Geometry: final body of the model. Coordinates: model frame, mm. A direction names the side the tool comes from. Round coordinates to 2 decimals unless told otherwise and drop trailing zeros. Loops run counter-clockwise (first coordinate to the right, second up) from the corner with the lowest first, then second, coordinate; pieces in that order, holes last. Notation, with made-up numbers: (83, 37) - (125, 37) arc R28 ccw to (125, 55) - close; hole circle Ø11 at (16.5, 55). An arc over 180 degrees is marked (long way). Write item = value, one per line. Start each with the question number.
Item 1: Section D-D (z = 12). Return loops of the section in (x, y).
Item 2: First-contact query: pin 1 (2 mm diameter, centred on y = -29.5, z = 12, fed in from -X); pin 2 (9 mm diameter, centred on y = -0.5, z = -4, fed in from -X); pin 3 (1.5 mm diameter, centred on y = 29.5, z = -12, fed in from +X). Flat tips, straight axial feed; report the tip coordinate or a pass-through.
Item 3: Section A-A (x = -23). Return loops of the section in (y, z).
Item 4: Access query for faces 5 (the flat face through (-14, 6, 12)), 6 (the flat face through (0, 32.5, 0)), 7 (the cylindrical face through (28.5, 23.5, 0.1)). Directions: +Z, -Z, +X, -X, +Y, -Y. A direction counts if a zero-diameter tool reaches every point of the face in a straight line with its end or side. Return the directions, or none.
Item 5: Line query: line 1 (Z direction, x = -21, y = 5.5); line 2 (Z direction, x = -17, y = -29); line 3 (X direction, y = 19.5, z = -7.75). Output: solid intervals per line, ascending. Write a range as from..to.
Item 6: Draft query along Z for faces 1 (the cylindrical face through (-19.07, 5.66, -10.76)), 2 (the flat face through (-24, 0, 0)), 3 (the flat face through (-14, -29, -12)), 4 (the flat face through (0, 0, 15)). Return one class per face: pulls with the +Z half, pulls with the -Z half, needs draft (parallel to the pull), parting line crosses it, or undercut.
Item 7: Section C-C (y = -29.5). Return loops of the section in (x, z).
from build123d import *

# Parameters (mm, degrees)
BOSS_EXTRUDE1_DEPTH      = 15
BOSS_EXTRUDE1_DEPTH_BACK = 15
SKETCH1_W                = 48
SKETCH1_H                = 65
SKETCH2_R                = 1.25
CUT_EXTRUDE1_DEPTH       = 10
SKETCH4_R                = 9.5
SKETCH4_R_2              = 8
SKETCH4_R_3              = 3
BOSS_EXTRUDE3_DEPTH      = 1.5
CHAMFER2_SIZE            = 1.5
SKETCH5_R                = 3
BOSS_EXTRUDE4_DEPTH      = 6
CHAMFER2_OF_MIRROR1_SIZE = 1.5


with BuildPart() as part:
    # Sketch1 → Boss-Extrude1 (new, two sides: drawn at the far end of the back side and taken through both)
    with BuildSketch(Plane.XY.offset(-BOSS_EXTRUDE1_DEPTH_BACK)):
        Rectangle(SKETCH1_W, SKETCH1_H)
    extrude(amount=BOSS_EXTRUDE1_DEPTH + BOSS_EXTRUDE1_DEPTH_BACK)

    # Sketch2 → Cut-Extrude1 (cut)
    with BuildSketch(Plane.ZY.offset(24)):
        with Locations(Location((-12, 29.5, 0), (0, 0, 270))):
            Circle(SKETCH2_R)
        with Locations(Location((12, 29.5, 0), (0, 0, 270))):
            Circle(SKETCH2_R)
        with Locations(Location((12, 5.5, 0), (0, 0, 270))):
            Circle(SKETCH2_R)
        with Locations(Location((-12, 5.5, 0), (0, 0, 270))):
            Circle(SKETCH2_R)
        with Locations(Location((-12, -29.5, 0), (0, 0, 270))):
            Circle(SKETCH2_R)
        with Locations(Location((12, -29.5, 0), (0, 0, 270))):
            Circle(SKETCH2_R)
    extrude(amount=-CUT_EXTRUDE1_DEPTH, mode=Mode.SUBTRACT)

    # Sketch4 → Boss-Extrude3 (add)
    # profile 1 of 3: a face of its own
    with BuildSketch(Plane.ZY.offset(24)):
        with Locations(Location((0, 20.5, 0), (0, 0, 270))):
            Circle(SKETCH4_R)
        with Locations((0, 20.5)):
            Circle(SKETCH4_R_2, mode=Mode.SUBTRACT)
    # profile 2 of 3: a face of its own
    with BuildSketch(Plane.ZY.offset(24)):
        with Locations((0, 20.5)):
            Circle(SKETCH4_R_2)
        with Locations((0, 20.5)):
            Circle(SKETCH4_R_3, mode=Mode.SUBTRACT)
    # profile 3 of 3: a face of its own
    with BuildSketch(Plane.ZY.offset(24)):
        with Locations((0, 20.5)):
            Circle(SKETCH4_R_3)
    boss_extrude3 = extrude(amount=BOSS_EXTRUDE3_DEPTH)

    # Chamfer2
    chamfer2_edges = [part.edges().sort_by_distance(p)[0] for p in [
        (-25.5, 30, 0),
    ]]
    chamfer(chamfer2_edges, length=CHAMFER2_SIZE - 0.0001)  # a hair under: the kernel refuses the full size

    # Sketch5 → Boss-Extrude4 (add)
    with BuildSketch(Plane.ZY.offset(25.5)):
        with Locations(Location((0, 20.5, 0), (0, 0, 270))):
            Circle(SKETCH5_R)
    boss_extrude4 = extrude(amount=BOSS_EXTRUDE4_DEPTH)

    # Mirror1: Boss-Extrude3, Boss-Extrude4 across plane
    add(boss_extrude3.mirror(Plane(origin=(0, 0, 0), x_dir=(0, 0, 1), z_dir=(1, 0, 0))))
    add(boss_extrude4.mirror(Plane(origin=(0, 0, 0), x_dir=(0, 0, 1), z_dir=(1, 0, 0))))

    # Chamfer2 of Mirror1
    chamfer2_of_mirror1_edges = [part.edges().sort_by_distance(p)[0] for p in [
        (25.5, 30, 0),
    ]]
    chamfer(chamfer2_of_mirror1_edges, length=CHAMFER2_OF_MIRROR1_SIZE - 0.0001)  # a hair under: the kernel refuses the full size


solid = part.part
Taken from the geometry:
q1.outline = (-24, -32.5) - (24, -32.5) - (24, 32.5) - (-24, 32.5) - (-24, 30.75) - (-14, 30.75) - (-14, 28.25) - (-24, 28.25) - (-24, 6.75) - (-14, 6.75) - (-14, 4.25) - (-24, 4.25) - (-24, -28.25) - (-14, -28.25) - (-14, -30.75) - (-24, -30.75) - close
q2.pin_1 = -14
q2.pin_2 = -24
q2.pin_3 = 24
q3.outline = (-32.5, -15) - (32.5, -15) - (32.5, 15) - (-32.5, 15) - close; hole circle Ø2.5 at (-29.5, -12); hole circle Ø2.5 at (-29.5, 12); hole circle Ø2.5 at (5.5, -12); hole circle Ø2.5 at (5.5, 12); hole circle Ø2.5 at (29.5, -12); hole circle Ø2.5 at (29.5, 12)
q4.face_5 = -X
q4.face_6 = +Z, -Z, +X, -X, +Y
q4.face_7 = +X
q5.line_1 = -15..-13.25, -10.75..10.75, 13.25..15
q5.line_2 = -15..-13.15, -10.85..10.85, 13.15..15
q5.line_3 = -25.5..25.5
q6.face_1 = undercut
q6.face_2 = needs draft
q6.face_3 = undercut
q6.face_4 = pulls with the +Z half
q7.outline = (-24, -15) - (24, -15) - (24, 15) - (-24, 15) - (-24, 13.25) - (-14, 13.25) - (-14, 10.75) - (-24, 10.75) - (-24, -10.75) - (-14, -10.75) - (-14, -13.25) - (-24, -13.25) - close
